from build123d import *

# Parameters (mm, degrees)
BOSS_EXTRUDE1_DEPTH     = 40
MOVE_FACE1_DEPTH        = 40
SKETCH2_OUTSIDE_W       = 54.614
SKETCH2_OUTSIDE_H       = 54.614
SKETCH2_OUTSIDE_W_2     = 40
SKETCH2_OUTSIDE_H_2     = 20
CUT_EXTRUDE1_DEPTH      = 51.372492072
SKETCH3_R               = 10
CUT_EXTRUDE2_DEPTH      = 15
CUT_EXTRUDE3_REACH      = 78.837
CUT_EXTRUDE3_END_RADIUS = 10
SKETCH4_R               = 2
SKETCH5_R               = 2
CUT_EXTRUDE4_DEPTH      = 51.372492116
SKETCH6_R               = 4
CUT_EXTRUDE5_DEPTH      = 4
SKETCH7_OUTSIDE_W       = 54.614
SKETCH7_OUTSIDE_H       = 54.614
SKETCH7_OUTSIDE_R       = 12
CUT_EXTRUDE6_DEPTH      = 18
SKETCH8_R               = 2.5
CUT_EXTRUDE9_DEPTH      = 49.758465533
SKETCH9_R               = 4.75
CUT_EXTRUDE10_DEPTH     = 2


# Read off the part's stored shape, not the designer's step: Move Face1
with BuildPart() as part:
    # Sketch1 → Boss-Extrude1 (new body)
    with BuildSketch(Plane.XY):
        Polygon((-15.872908622, 29.998965851), (-14.072908622, 28.198965851), (-16.792908622, 28.198965851), (-16.792908622, 26.558965851), (-14.132908622, 23.898965851), (-8.452908622, 23.898965851), (-5.792908622, 26.558965851), (-5.792908622, 28.198965851), (-8.512908622, 28.198965851), (-6.712908622, 29.998965851), (4.127091378, 29.998965851), (5.927091378, 28.198965851), (3.207091378, 28.198965851), (3.207091378, 26.558965851), (5.867091378, 23.898965851), (11.547091378, 23.898965851), (14.207091378, 26.558965851), (14.207091378, 28.198965851), (11.487091378, 28.198965851), (13.287091378, 29.998965851), (18.707091378, 29.998965851), (18.707091378, 51.998965851), (-21.292908622, 51.998965851), (-21.292908622, 29.998965851), align=None)
    extrude(amount=BOSS_EXTRUDE1_DEPTH)

    # Move Face1 outline → Move Face1 (cut)
    with BuildSketch(Plane.XY):
        Polygon((-16.592908622, 27.998965851), (-13.590065909, 27.998965851), (-15.590065909, 29.998965851), (-15.872908622, 29.998965851), (-14.072908622, 28.198965851), (-16.792908622, 28.198965851), (-16.792908622, 26.558965851), (-14.132908622, 23.898965851), (-8.452908622, 23.898965851), (-5.792908622, 26.558965851), (-5.792908622, 28.198965851), (-8.512908622, 28.198965851), (-6.712908622, 29.998965851), (-6.995751334, 29.998965851), (-8.995751334, 27.998965851), (-5.992908622, 27.998965851), (-5.992908622, 26.641808564), (-8.535751334, 24.098965851), (-14.050065909, 24.098965851), (-16.592908622, 26.641808564), align=None)
        Polygon((4.409934091, 29.998965851), (4.127091378, 29.998965851), (5.927091378, 28.198965851), (3.207091378, 28.198965851), (3.207091378, 26.558965851), (5.867091378, 23.898965851), (11.547091378, 23.898965851), (14.207091378, 26.558965851), (14.207091378, 28.198965851), (11.487091378, 28.198965851), (13.287091378, 29.998965851), (13.004248666, 29.998965851), (11.004248666, 27.998965851), (14.007091378, 27.998965851), (14.007091378, 26.641808564), (11.464248666, 24.098965851), (5.949934091, 24.098965851), (3.407091378, 26.641808564), (3.407091378, 27.998965851), (6.409934091, 27.998965851), align=None)
    extrude(amount=MOVE_FACE1_DEPTH, mode=Mode.SUBTRACT)

    # Sketch2 outside → Cut-Extrude1 (cut, through all)
    with BuildSketch(Plane.XZ.offset(-29.998965851)):
        with Locations((-1.293, 20)):
            Rectangle(SKETCH2_OUTSIDE_W, SKETCH2_OUTSIDE_H)
        with Locations((-1.292908622, 20)):
            Rectangle(SKETCH2_OUTSIDE_W_2, SKETCH2_OUTSIDE_H_2, mode=Mode.SUBTRACT)
    extrude(amount=CUT_EXTRUDE1_DEPTH, mode=Mode.SUBTRACT)

    # Sketch3 → Cut-Extrude2 (cut)
    with BuildSketch(Plane(origin=(0, 51.998965851, 0), x_dir=(1, 0, 0), z_dir=(0, 1, 0))):
        with Locations(Location((-1.292908622, -20, 0), (0, 0, 270))):
            Circle(SKETCH3_R)
    extrude(amount=-CUT_EXTRUDE2_DEPTH, mode=Mode.SUBTRACT)

    # Cut-Extrude3: up to this cylinder (the profile starts outside it)
    cut_extrude3_end = Plane(origin=(-1.292908622, 38.998966, 20), z_dir=(0, 1, 0)) * Cylinder(CUT_EXTRUDE3_END_RADIUS, 178.674, mode=Mode.PRIVATE)
    # Sketch4 → Cut-Extrude3 (cut, up to the surface)
    with BuildSketch(Plane(origin=(18.707091378, 0, 0), x_dir=(0, 0, -1), z_dir=(1, 0, 0)), mode=Mode.PRIVATE) as cut_extrude3_sk1:
        with Locations(Location((-20, 38.998965851, 0), (0, 0, 90))):
            Circle(SKETCH4_R)
    cut_extrude3_tool1 = extrude(cut_extrude3_sk1.sketch, amount=-CUT_EXTRUDE3_REACH, mode=Mode.PRIVATE) - cut_extrude3_end
    add(cut_extrude3_tool1.solids().sort_by_distance((18.707091, 38.998966, 20))[0], mode=Mode.SUBTRACT)

    # Sketch5 → Cut-Extrude4 (cut, through all)
    with BuildSketch(Plane.XZ.offset(-29.998965851)):
        with Locations((-1.292908622, 20)):
            Circle(SKETCH5_R)
    extrude(amount=-CUT_EXTRUDE4_DEPTH, mode=Mode.SUBTRACT)

    # Sketch6 → Cut-Extrude5 (cut)
    with BuildSketch(Plane.XZ.offset(-29.998965851)):
        with Locations((-1.292908622, 20)):
            Circle(SKETCH6_R)
    extrude(amount=-CUT_EXTRUDE5_DEPTH, mode=Mode.SUBTRACT)

    # Sketch7 outside → Cut-Extrude6 (cut)
    with BuildSketch(Plane(origin=(0, 51.998965851, 0), x_dir=(1, 0, 0), z_dir=(0, 1, 0))):
        with Locations((-1.293, -20)):
            Rectangle(SKETCH7_OUTSIDE_W, SKETCH7_OUTSIDE_H)
        with Locations(Location((-1.292908622, -20, 0), (0, 0, 270))):
            Circle(SKETCH7_OUTSIDE_R, mode=Mode.SUBTRACT)
    extrude(amount=-CUT_EXTRUDE6_DEPTH, mode=Mode.SUBTRACT)

    # Sketch8 → Cut-Extrude9 (cut, through all)
    with BuildSketch(Plane(origin=(0, 33.998965851, 0), x_dir=(1, 0, 0), z_dir=(0, 1, 0))):
        with Locations(Location((8.707091378, -5, 0), (0, 0, 270))):
            Circle(SKETCH8_R)
        with Locations(Location((-11.292908622, -5, 0), (0, 0, 270))):
            Circle(SKETCH8_R)
        with Locations(Location((-11.292908622, -35, 0), (0, 0, 270))):
            Circle(SKETCH8_R)
        with Locations(Location((8.707091378, -35, 0), (0, 0, 270))):
            Circle(SKETCH8_R)
    extrude(amount=-CUT_EXTRUDE9_DEPTH, mode=Mode.SUBTRACT)

    # Sketch9 → Cut-Extrude10 (cut)
    with BuildSketch(Plane(origin=(0, 33.998965851, 0), x_dir=(1, 0, 0), z_dir=(0, 1, 0))):
        with Locations(Location((8.707091378, -5, 0), (0, 0, 270))):
            Circle(SKETCH9_R)
        with Locations(Location((8.707091378, -35, 0), (0, 0, 270))):
            Circle(SKETCH9_R)
        with Locations(Location((-11.292908622, -35, 0), (0, 0, 270))):
            Circle(SKETCH9_R)
        with Locations(Location((-11.292908622, -5, 0), (0, 0, 270))):
            Circle(SKETCH9_R)
    extrude(amount=-CUT_EXTRUDE10_DEPTH, mode=Mode.SUBTRACT)


solid = part.part
Could you check a few things on this model? Use its own coordinates, in mm. A direction names the side the tool comes from. Coordinates: 2 decimals unless noted, no trailing zeros. Loops run counter-clockwise (first coordinate to the right, second up) from the corner with the lowest first, then second, coordinate; pieces in that order, holes last. Notation, with made-up numbers: (-24.5, 55) -> (4.5, 55) arc R17 ccw to (4.5, 67) -> close; hole circle Ø9 at (5, 27.25). An arc over 180 degrees is marked (long way). Answer in a Markdown table with one row per item.
(1) Imagine slicing it at A-A (z = 5). List the corners of the cut face in (x, y) for me, plus the area to 3 significant figures.
Results found:
| item | result |
|---|---|
| outline | (-21.29, 30) -> (-13.79, 30) -> (-13.79, 32) -> (-16.04, 32) -> (-16.04, 34) -> (-21.29, 34) -> close; (-8.79, 30) -> (6.21, 30) -> (6.21, 32) -> (3.96, 32) -> (3.96, 34) -> (-6.54, 34) -> (-6.54, 32) -> (-8.79, 32) -> close; (11.21, 30) -> (18.71, 30) -> (18.71, 34) -> (13.46, 34) -> (13.46, 32) -> (11.21, 32) -> close |
| area | 102 mm^2 |
(2) Imagine slicing it at C-C (z = 38.5). List the corners of the cut face in (x, y) for me.
Results found:
| item | result |
|---|---|
| outline | (-21.29, 30) -> (18.71, 30) -> (18.71, 34) -> (11.92, 34) -> (11.92, 32) -> (5.5, 32) -> (5.5, 34) -> (-8.08, 34) -> (-8.08, 32) -> (-14.5, 32) -> (-14.5, 34) -> (-21.29, 34) -> close |
(3) If I drill on probe 1 along X at (y, z) = (33, 35); probe 2 along Y at (x, z) = (9.5, 20.5); probe 3 along Z at (x, y) = (4.5, 50.5), over which ranges is the centre line in solid material (lowest first)?
Results found:
| item | result |
|---|---|
| probe 1 | x = -21.29 to -16.04, -6.54 to 3.96, 13.46 to 18.71 |
| probe 2 | y = 24.1 to 37.06, 40.94 to 52 |
| probe 3 | z = 9.49 to 11.85, 28.15 to 30.51 |
(4) Will these pins go through, and if not, where does the flat tip stop? pin 1 Ø6.5 at (x, y) = (-9.5, 26.5) entering from +Z; pin 2 Ø4 at (x, z) = (-17, 19.5) entering from +Y; pin 3 Ø1.5 at (y, z) = (27.5, 22) entering from +X; pin 4 Ø6 at (x, y) = (8.5, 33) entering from -Z.
Results found:
| item | result |
|---|---|
| pin 1 | stops at z = 30 |
| pin 2 | stops at y = 34 |
| pin 3 | stops at x = 14.01 |
| pin 4 | stops at z = 0 |
(5) Imagine slicing it at B-B (x = 8). Give the number of separate pieces and of enclosed holes in the cut face, plus the area to 3 significant figures.
Results found:
| item | result |
|---|---|
| separate pieces | 3 |
| enclosed holes | 0 |
| area | 384 mm^2 |
(6) For faces 1 (the face through (9, 27, 30)), 2 (the face through (-1.814, 31.971, 23.966)), 3 (the face through (-16.593, 27, 20)), 4 (the face through (-11, 27, 10)), which set-ups out of +Z, -Z, +X, -X, +Y, -Y let a thin tool reach every point of the face, with its end or its side?
Results found:
| item | result |
|---|---|
| face 1 | +Z, +X, -X, -Y |
| face 2 | -Y |
| face 3 | +Z, -Z, -X, -Y |
| face 4 | -Z, +X, -X, -Y |
(7) Thinking about a two-plate mould opening in Y: for faces 5 (the face through (-8, 27.999, 20)), 6 (the face through (-13.3, 31.999, 37)), 7 (the face through (-1.553, 35.478, 21.983)), 8 (the face through (5.424, 28.985, 19.86)), which applies, released by +Y, released by -Y, zero draft, split by the parting line, or undercut?
Results found:
| item | result |
|---|---|
| face 5 | undercut |
| face 6 | released by +Y |
| face 7 | zero draft |
| face 8 | undercut |
(8) Imagine slicing it at D-D (x = -4). List the corners of the cut face in (y, z) for me.
Results found:
| item | result |
|---|---|
| outline | (30, 0) -> (34, 0) -> (34, 8.31) -> (52, 8.31) -> (52, 10.37) -> (37, 10.37) -> (37, 29.63) -> (52, 29.63) -> (52, 31.69) -> (34, 31.69) -> (34, 40) -> (30, 40) -> (30, 22.94) -> (34, 22.94) -> (34, 17.06) -> (30, 17.06) -> close |
